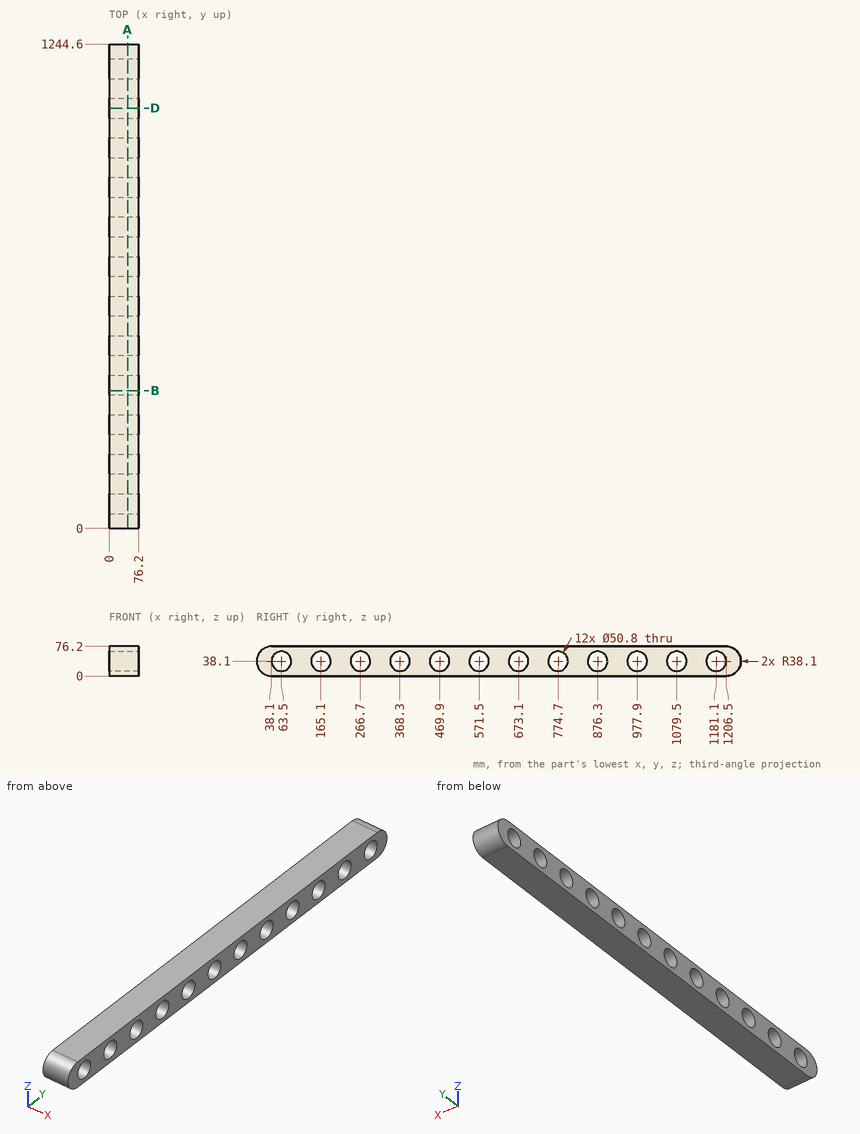
Print and shaded views of the part. All mm, measured from the part's lowest x, y and z. Coordinates: 2 decimals unless noted, no trailing zeros. Order: outer loops, then holes, each group sorted by start corner. A loop starts at its lowest first (then second) coordinate and runs counter-clockwise, first axis right, second up. Notation, with made-up numbers: (-24, 80) -> (10, 80) arc R18 ccw to (10, 92) -> close; hole circle Ø6 at (2.25, 59.25). An arc over 180 degrees is marked (long way). Answer as a JSON object with one key per item and string values. Group by question number.
1) Cut at B-B, the plane y = 354. Write the cut outline in (x, z).
2) Cut at D-D, the plane y = 1079.5. Write the cut outline in (x, z).
3) Cut at A-A, the plane x = 48. Count the separate pieces of the cut face and the enclosed holes in it, then the cut area to 3 significant figures.
4) Drill centre lines: L1, parallel to Z at x = 11.5, y = 167; L2, parallel to Z at x = 58, y = 876; L3, parallel to Y at x = 36, z = 65. Where is each one in solid material? Low to high.
5) Flat gauge pin, fed straight in: pin 1 (4 mm diameter, centred on x = 11, y = 178, fed in from -Z). Where does the tip first touch, or does it go through?
Check values:
{
 "1": {"outline": "(0, 0) -> (76.2, 0) -> (76.2, 17.11) -> (0, 17.11) -> close; (0, 59.09) -> (76.2, 59.09) -> (76.2, 76.2) -> (0, 76.2) -> close"},
 "2": {"outline": "(0, 0) -> (76.2, 0) -> (76.2, 12.7) -> (0, 12.7) -> close; (0, 63.5) -> (76.2, 63.5) -> (76.2, 76.2) -> (0, 76.2) -> close"},
 "3": {"separate pieces": "1", "enclosed holes": "12", "area": "69,300 mm²"},
 "4": {"L1": "z = 0 to 12.77, 63.43 to 76.2", "L2": "z = 0 to 12.7, 63.5 to 76.2", "L3": "y = 11.12 to 1233.48"},
 "5": {"pin 1": "stops at z = 0"}
}
